Could you check a few things on this model? Use its own coordinates, in mm. Give positions to 0.01 mm unless a question says otherwise; leave off trailing zeros. Loops run counter-clockwise (first coordinate to the right, second up) from the corner with the lowest first, then second, coordinate; pieces in that order, holes last. Notation, with made-up numbers: M -21.5,-18.75 L -3.5,-18.75 A19 cw -3.5,12.25 Z; hole C 52.5,73 d2. An arc over 180 degrees is marked long. Use a Markdown table: item, result. Add a question column.
1) Suppose I cut it at C-C on x = -9. List the corners of the cut face in (y, z) for me.
2) Suppose I cut it at B-B on y = -2.4. List the corners of the cut face in (x, z) for me, and give its area (3 significant figures).
3) Suppose I cut it at A-A on z = 0. List the corners of the cut face in (x, y) for me, and give its area (3 significant figures).
4) If I drill on line 1 along X through (y, z) = (-3.4, -45); line 2 along Z through (x, y) = (44.5, -1); line 3 along Z through (x, y) = (19.5, -3.3), over which ranges is the centre line in solid material (lowest first)? Write a range as [from, to].
5) We'd pull the mould along X, two halves only. Please class faces 1 (the cylindrical face through (27.204, -1.932, -48.794)), 2 (the flat face through (-63.5, -2, -1)), 3 (the flat face through (-1, -2, -71.12)): +X half, -X half, draft (parallel to the pull), parting line (faces both ways), or undercut.
```python
from build123d import *

# Parameters (mm, degrees)
F0_W     = 127
F0_H     = 142.24
F1_DEPTH = 3.81
F2_R     = 55
F3_DEPTH = 3.81
F5_DEPTH = 3.81


with BuildPart() as f1:
    # F0 (on Front) → F1 (new body)
    with BuildSketch(Plane.XZ):
        Rectangle(F0_W, F0_H)
    extrude(amount=F1_DEPTH)

    # F2 (on face) → F3 (cut, through all)
    with BuildSketch(Plane.XZ.offset(3.81)):
        with Locations((1.824845, 0)):
            Circle(F2_R)
    extrude(amount=-F3_DEPTH, mode=Mode.SUBTRACT)

    # F4 (on face) → F5 (cut, through all)
    with BuildSketch(Plane.XZ.offset(3.81)):
        with BuildLine():
            ThreePointArc((-46.463834, 43.282353), (-44.881349, 42.651369), (-43.31029, 43.31029))
            Line((-43.31029, 43.31029), (-44.901281, 44.901281))
            ThreePointArc((-44.901281, 44.901281), (-45.689728, 44.098738), (-46.463834, 43.282353))
        make_face()
        with BuildLine():
            ThreePointArc((-44.901281, 44.901281), (-44.098738, 45.689728), (-43.282353, 46.463834))
            ThreePointArc((-43.282353, 46.463834), (-46.492271, 46.492271), (-46.463834, 43.282353))
            ThreePointArc((-46.463834, 43.282353), (-45.689728, 44.098738), (-44.901281, 44.901281))
        make_face()
        with BuildLine():
            ThreePointArc((-42.651281, 44.901281), (-42.815006, 45.74387), (-43.282353, 46.463834))
            ThreePointArc((-43.282353, 46.463834), (-44.098738, 45.689728), (-44.901281, 44.901281))
            Line((-44.901281, 44.901281), (-43.31029, 43.31029))
            ThreePointArc((-43.31029, 43.31029), (-42.822552, 44.040243), (-42.651281, 44.901281))
        make_face()
        with BuildLine():
            ThreePointArc((44.901281, 44.901281), (45.689728, 44.098738), (46.463834, 43.282353))
            ThreePointArc((46.463834, 43.282353), (46.9723, 44.021862), (47.151281, 44.901281))
            ThreePointArc((47.151281, 44.901281), (45.74387, 46.987556), (43.282353, 46.463834))
            ThreePointArc((43.282353, 46.463834), (44.098738, 45.689728), (44.901281, 44.901281))
        make_face()
        with BuildLine():
            ThreePointArc((43.31029, 43.31029), (44.881349, 42.651369), (46.463834, 43.282353))
            ThreePointArc((46.463834, 43.282353), (45.689728, 44.098738), (44.901281, 44.901281))
            Line((44.901281, 44.901281), (43.31029, 43.31029))
        make_face()
        with BuildLine():
            Line((43.31029, 43.31029), (44.901281, 44.901281))
            ThreePointArc((44.901281, 44.901281), (44.098738, 45.689728), (43.282353, 46.463834))
            ThreePointArc((43.282353, 46.463834), (42.651369, 44.881349), (43.31029, 43.31029))
        make_face()
        with BuildLine():
            ThreePointArc((44.901281, -44.901281), (45.689728, -44.098738), (46.463834, -43.282353))
            ThreePointArc((46.463834, -43.282353), (44.881349, -42.651369), (43.31029, -43.31029))
            Line((43.31029, -43.31029), (44.901281, -44.901281))
        make_face()
        with BuildLine():
            ThreePointArc((43.282353, -46.463834), (44.098738, -45.689728), (44.901281, -44.901281))
            Line((44.901281, -44.901281), (43.31029, -43.31029))
            ThreePointArc((43.31029, -43.31029), (42.651369, -44.881349), (43.282353, -46.463834))
        make_face()
        with BuildLine():
            ThreePointArc((47.151281, -44.901281), (46.9723, -44.021862), (46.463834, -43.282353))
            ThreePointArc((46.463834, -43.282353), (45.689728, -44.098738), (44.901281, -44.901281))
            ThreePointArc((44.901281, -44.901281), (44.098738, -45.689728), (43.282353, -46.463834))
            ThreePointArc((43.282353, -46.463834), (45.74387, -46.987556), (47.151281, -44.901281))
        make_face()
        with BuildLine():
            ThreePointArc((-46.463834, -43.282353), (-46.492271, -46.492271), (-43.282353, -46.463834))
            ThreePointArc((-43.282353, -46.463834), (-44.098738, -45.689728), (-44.901281, -44.901281))
            ThreePointArc((-44.901281, -44.901281), (-45.689728, -44.098738), (-46.463834, -43.282353))
        make_face()
        with BuildLine():
            Line((-44.901281, -44.901281), (-43.31029, -43.31029))
            ThreePointArc((-43.31029, -43.31029), (-44.881349, -42.651369), (-46.463834, -43.282353))
            ThreePointArc((-46.463834, -43.282353), (-45.689728, -44.098738), (-44.901281, -44.901281))
        make_face()
        with BuildLine():
            ThreePointArc((-42.651281, -44.901281), (-42.822552, -44.040243), (-43.31029, -43.31029))
            Line((-43.31029, -43.31029), (-44.901281, -44.901281))
            ThreePointArc((-44.901281, -44.901281), (-44.098738, -45.689728), (-43.282353, -46.463834))
            ThreePointArc((-43.282353, -46.463834), (-42.815006, -45.74387), (-42.651281, -44.901281))
        make_face()
    extrude(amount=-F5_DEPTH, mode=Mode.SUBTRACT)


solid = f1.part
```
Answer block:
| question | item | result |
|---|---|---|
| 1 | outline | M -3.81,-71.12 L 0,-71.12 L 0,-53.92 L -3.81,-53.92 Z; M -3.81,53.92 L 0,53.92 L 0,71.12 L -3.81,71.12 Z |
| 2 | outline | M -63.5,-71.12 L 63.5,-71.12 L 63.5,71.12 L -63.5,71.12 Z; hole C 1.82,0 d110; hole M -46.46,-43.28 A2.25 ccw long -42.65,-44.9 A2.25 ccw -43.31,-43.31 A2.25 ccw Z; hole M -46.46,43.28 A2.25 ccw -43.31,43.31 A2.25 ccw -42.65,44.9 A2.25 ccw long Z; hole M 43.28,-46.46 A2.25 ccw 47.15,-44.9 A2.25 ccw 46.46,-43.28 A2.25 ccw 43.31,-43.31 A2.25 ccw Z; hole M 43.28,46.46 A2.25 ccw 43.31,43.31 A2.25 ccw 46.46,43.28 A2.25 ccw 47.15,44.9 A2.25 ccw Z |
| 2 | area | 8,500 mm^2 |
| 3 | outline | M -63.5,-3.81 L -53.18,-3.81 L -53.18,0 L -63.5,0 Z; M 56.82,-3.81 L 63.5,-3.81 L 63.5,0 L 56.82,0 Z |
| 3 | area | 64.8 mm^2 |
| 4 | line 1 | x = [-63.5, -47.15], [-42.65, -29.8], [33.45, 42.65], [47.15, 63.5] |
| 4 | line 2 | z = [-71.12, -47.12], [-42.69, -34.7], [34.7, 42.69], [47.12, 71.12] |
| 4 | line 3 | z = [-71.12, -52.08], [52.08, 71.12] |
| 5 | face 1 | undercut |
| 5 | face 2 | -X half |
| 5 | face 3 | draft |
